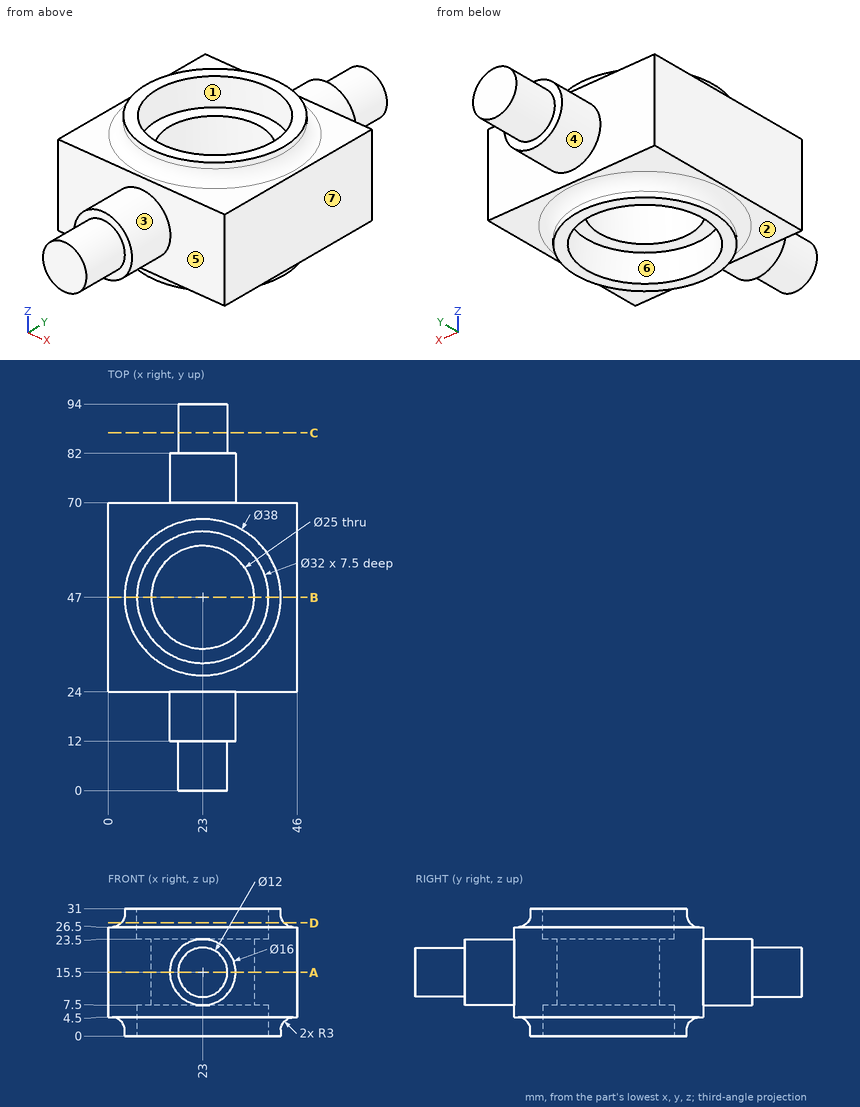
Answer from the drawing. Dimensions are ordinates in mm from the lowest x, y and z of the part. A direction names the side the tool comes from. Coordinates: 2 decimals unless noted, no trailing zeros. Write each loop counter-clockwise with the first axis right and the second up, starting at its lowest first coordinate (ties: lowest second). Pieces come first, ordered by that corner, then holes. Notation, with made-up numbers: M 70.25,-18 L 126.25,-18 A29 ccw 126.25,17 Z; hole C -8,15 d1. An arc over 180 degrees is marked long. Use a Markdown table: item, result.
Q1. The part is cut by section D-D, the plane z = 27.5. Write down the section's boundary in (x, y).
Answer block:
| item | result |
|---|---|
| outline | C 23,47 d39.53; hole C 23,47 d32 |
Q2. Each of these flat-tipped pins is pushed along its axis until it touches: pin 1 Ø16 at (x, y) = (26.5, 40.5) entering from +Z; pin 2 Ø10 at (x, z) = (19.5, 26) entering from -Y; pin 3 Ø1 at (x, y) = (27, 26) entering from -Z. Where does it stop, or does it pass through?
Answer block:
| item | result |
|---|---|
| pin 1 | stops at z = 23.5 |
| pin 2 | stops at y = 12 |
| pin 3 | stops at z = 4.28 |
Q3. The part is cut by section A-A, the plane z = 15.5. Write down the section's boundary in (x, y).
Answer block:
| item | result |
|---|---|
| outline | M 0,24 L 15,24 L 15,12 L 17,12 L 17,0 L 29,0 L 29,12 L 31,12 L 31,24 L 46,24 L 46,70 L 31,70 L 31,82 L 29,82 L 29,94 L 17,94 L 17,82 L 15,82 L 15,70 L 0,70 Z; hole C 23,47 d25 |
Q4. The part is cut by section C-C, the plane y = 87. Write down the section's boundary in (x, z).
Answer block:
| item | result |
|---|---|
| outline | C 23,15.5 d12 |
Q5. The part is cut by section B-B, the plane y = 47. Write down the section's boundary in (x, z).
Answer block:
| item | result |
|---|---|
| outline | M 0,4.5 L 1,4.5 A3 cw 4,1.5 L 4,0 L 7,0 L 7,7.5 L 10.5,7.5 L 10.5,23.5 L 7,23.5 L 7,31 L 4,31 L 4,29.5 A3 cw 1,26.5 L 0,26.5 Z; M 35.5,7.5 L 39,7.5 L 39,0 L 42,0 L 42,1.5 A3 cw 45,4.5 L 46,4.5 L 46,26.5 L 45,26.5 A3 cw 42,29.5 L 42,31 L 39,31 L 39,23.5 L 35.5,23.5 Z |
Q6. Straight lines are drawn through the part: L1, parallel to Y at x = 23, z = 11; L2, parallel to Y at x = 23, z = 26; L3, parallel to X at y = 80, z = 15. For each, find the intervals that lie inside material, in ascending order. Write a range as [from, to].
Answer block:
| item | result |
|---|---|
| L1 | y = [0, 34.5], [59.5, 94] |
| L2 | y = [24, 31], [63, 70] |
| L3 | x = [15.02, 30.98] |
Q7. Which of the six approach directions +Z, -Z, +X, -X, +Y, -Y give full straight-line access (tool end or side, diameter ignored) to the marked faces 1, 2, 3 and 4?
Answer block:
| item | result |
|---|---|
| face 1 | +Z |
| face 2 | -Z |
| face 3 | -Y |
| face 4 | +Y |
Q8. Determine the mould class of the marked faces 5, 6 and 7 for opening direction X: released by +X, released by -X, zero draft, split by the parting line, or undercut.
Answer block:
| item | result |
|---|---|
| face 5 | zero draft |
| face 6 | undercut |
| face 7 | released by +X |
